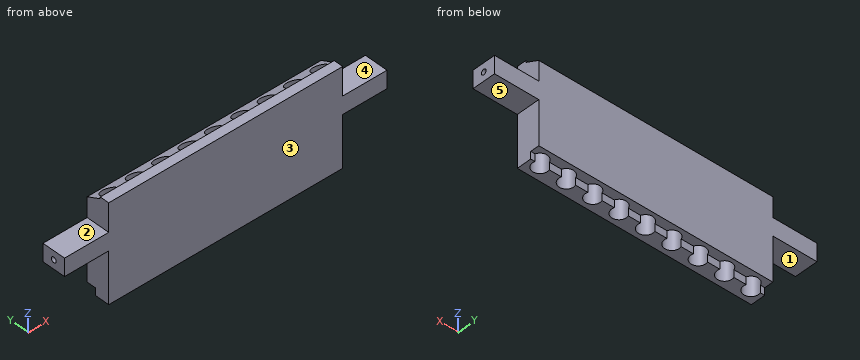
```python
from build123d import *

# Parameters (mm, degrees)
SKETCH_1_W          = 220
SKETCH_1_H          = 16
SKETCH_1_R          = 5.1
EXTRUDE_1_DEPTH     = 65
SKETCH_2_W          = 220
SKETCH_2_H          = 5
CUT_EXTRUDE_1_DEPTH = 6
SKETCH_3_W          = 30.147927972
SKETCH_3_H          = 35
SKETCH_3_H_2        = 18
SKETCH_3_W_2        = 30.207927972
CUT_EXTRUDE_2_DEPTH = 230.958691943
SKETCH_4_R          = 1.8
CUT_EXTRUDE_3_DEPTH = 10
CUT_EXTRUDE_START   = -10
SKETCH_5_R          = 1.8
CUT_EXTRUDE_4_DEPTH = 10
CUT_EXTRUDE_7_DEPTH = 202.251162989
SKETCH_9_W          = 159.644144056
SKETCH_9_H          = 6.33180748
EXTRUDE_2_DEPTH     = 1.2


with BuildPart() as part:
    # Эскиз1 → Бобышка-Вытянуть1 (new body)
    with BuildSketch(Plane.XY):
        with Locations((110, 8)):
            Rectangle(SKETCH_1_W, SKETCH_1_H)
        with Locations((37.97, 8.339391268)):
            Circle(SKETCH_1_R, mode=Mode.SUBTRACT)
        with Locations((55.97, 8.339391268)):
            Circle(SKETCH_1_R, mode=Mode.SUBTRACT)
        with Locations((73.97, 8.339391268)):
            Circle(SKETCH_1_R, mode=Mode.SUBTRACT)
        with Locations((91.97, 8.339391268)):
            Circle(SKETCH_1_R, mode=Mode.SUBTRACT)
        with Locations((109.97, 8.339391268)):
            Circle(SKETCH_1_R, mode=Mode.SUBTRACT)
        with Locations((127.97, 8.339391268)):
            Circle(SKETCH_1_R, mode=Mode.SUBTRACT)
        with Locations((145.97, 8.339391268)):
            Circle(SKETCH_1_R, mode=Mode.SUBTRACT)
        with Locations((163.97, 8.339391268)):
            Circle(SKETCH_1_R, mode=Mode.SUBTRACT)
        with Locations((181.97, 8.339391268)):
            Circle(SKETCH_1_R, mode=Mode.SUBTRACT)
    extrude(amount=EXTRUDE_1_DEPTH)

    # Эскиз2 → Вырез-Вытянуть1 (cut)
    with BuildSketch(Plane(origin=(0, 16, 0), x_dir=(1, 0, 0), z_dir=(0, 1, 0))):
        with Locations((110, -2.5)):
            Rectangle(SKETCH_2_W, SKETCH_2_H)
    extrude(amount=-CUT_EXTRUDE_1_DEPTH, mode=Mode.SUBTRACT)

    # Эскиз3 → Вырез-Вытянуть2 (cut, through all)
    with BuildSketch(Plane(origin=(0, 16, 0), x_dir=(1, 0, 0), z_dir=(0, 1, 0))):
        with Locations((15.073963986, -17.5)):
            Rectangle(SKETCH_3_W, SKETCH_3_H)
        with Locations((15.073963986, -56)):
            Rectangle(SKETCH_3_W, SKETCH_3_H_2)
        with Locations((204.896036014, -17.5)):
            Rectangle(SKETCH_3_W_2, SKETCH_3_H)
        with Locations((204.896036014, -56)):
            Rectangle(SKETCH_3_W_2, SKETCH_3_H_2)
    extrude(amount=-CUT_EXTRUDE_2_DEPTH, mode=Mode.SUBTRACT)

    # Эскиз4 → Вырез-Вытянуть3 (cut)
    with BuildSketch(Plane.ZY):
        with Locations((41, 8)):
            Circle(SKETCH_4_R)
    extrude(amount=-CUT_EXTRUDE_3_DEPTH, mode=Mode.SUBTRACT)

    # Эскиз5 → Вырез-Вытянуть4 (cut)
    with BuildSketch(Plane(origin=(220, 0, 0), x_dir=(0, 0, -1), z_dir=(1, 0, 0)).offset(CUT_EXTRUDE_START)):
        with Locations(Location((-41, 8, 0), (0, 0, 180))):
            Circle(SKETCH_5_R)
    extrude(amount=CUT_EXTRUDE_4_DEPTH, mode=Mode.SUBTRACT)

    # Эскиз8 → Вырез-Вытянуть7 (cut, through all)
    with BuildSketch(Plane(origin=(189.792072028, 0, 0), x_dir=(0, 0, -1), z_dir=(1, 0, 0))):
        Polygon((-65, 6.33180748), (-60.500350176, 16), (-65, 16), align=None)
    extrude(amount=-CUT_EXTRUDE_7_DEPTH, mode=Mode.SUBTRACT)

    # Эскиз9 → Бобышка-Вытянуть2 (add)
    with BuildSketch(Plane.XY.offset(65)):
        with Locations((109.97, 3.16590374)):
            Rectangle(SKETCH_9_W, SKETCH_9_H)
    extrude(amount=EXTRUDE_2_DEPTH)


solid = part.part
```
Can you work these out from the model? Positions are in its coordinate system, mm. Face numbers are marked on the shaded views. A direction names the side the tool comes from. Coordinates: 2 decimals unless noted, no trailing zeros. Loops run counter-clockwise (first coordinate to the right, second up) from the corner with the lowest first, then second, coordinate; pieces in that order, holes last. Notation, with made-up numbers: (-37.75, 7.25) - (3.25, 7.25) arc R20 ccw to (3.25, 15.25) - close; hole circle Ø7 at (48.5, -31). An arc over 180 degrees is marked (long way). Use a Markdown table: item, result.
Item 1: Will these pins go through, and if not, where does the flat tip stop? pin 1 (1 mm diameter, centred on y = 13, z = 53.5, fed in from -X); pin 2 (5 mm diameter, centred on y = 12, z = 59.5, fed in from +X); pin 3 (0.9 mm diameter, centred on x = 110.5, y = 4.5, fed in from -Z).
Numbers:
| item | result |
|---|---|
| pin 1 | stops at x = 30.15 |
| pin 2 | stops at x = 189.79 |
| pin 3 | stops at z = 65 |
Item 2: I want a section at D-D on x = 14.5. Please give me the cut outline in (y, z), and give its area (3 significant figures).
Numbers:
| item | result |
|---|---|
| outline | (0, 35) - (16, 35) - (16, 47) - (0, 47) - close |
| area | 192 mm2 |
Item 3: If I drill on probe 1 along Y at (x, z) = (212, 41); probe 2 along Y at (x, z) = (127.97, 27); probe 3 along Z at (x, y) = (215.75, 8), over which ranges is the centre line in solid material (lowest first)? Write a range as from..to.
Numbers:
| item | result |
|---|---|
| probe 1 | y = 0..6.2, 9.8..16 |
| probe 2 | y = 0..3.24, 13.44..16 |
| probe 3 | z = 35..39.2, 42.8..47 |
Item 4: I want a section at B-B on x = 145.97. Please give me the cut outline in (y, z), and give its area (3 significant figures).
Numbers:
| item | result |
|---|---|
| outline | (0, 0) - (3.24, 0) - (3.24, 65) - (6.33, 65) - (6.33, 66.2) - (0, 66.2) - close; (13.44, 5) - (16, 5) - (16, 60.5) - (13.44, 61.69) - close |
| area | 362 mm2 |
Item 5: I want a section at C-C on z = 54. Give the number of separate pieces and of enclosed holes in the cut face, and give its area (3 significant figures).
Numbers:
| item | result |
|---|---|
| separate pieces | 1 |
| enclosed holes | 9 |
| area | 1,820 mm2 |
Item 6: For the marked faces 1, 2, 3, 4 and 5, which set-ups out of +Z, -Z, +X, -X, +Y, -Y let a thin tool reach every point of the face, with its end or its side?
Numbers:
| item | result |
|---|---|
| face 1 | -Z, -X, +Y, -Y |
| face 2 | +Z, -X, +Y, -Y |
| face 3 | +Z, -Z, +X, -X, -Y |
| face 4 | +Z, +X, +Y, -Y |
| face 5 | -Z, +X, +Y, -Y |
Item 7: I want a section at A-A on x = 175. Please give me the cut outline in (y, z), and give its area (3 significant figures).
Numbers:
| item | result |
|---|---|
| outline | (0, 0) - (10, 0) - (10, 5) - (16, 5) - (16, 60.5) - (6.33, 65) - (6.33, 66.2) - (0, 66.2) - close |
| area | 996 mm2 |
